Can you work these out from the model? Positions are in its coordinate system, mm. A direction names the side the tool comes from. Give positions to 0.01 mm unless a question says otherwise; leave off trailing zeros. Order: outer loops, then holes, each group sorted by start corner. A loop starts at its lowest first (then second) coordinate and runs counter-clockwise, first axis right, second up. Notation, with made-up numbers: (-28.5, -22.5) - (16.5, -22.5) arc R13 ccw to (16.5, -6.5) - close; hole circle Ø10 at (50.5, 32.5). An arc over 180 degrees is marked (long way). Answer as CSV lines item,"result".
```python
from build123d import *

# Parameters (mm, degrees)
SKETCH_1_R          = 1
EXTRUDE_1_DEPTH     = 4
SKETCH_2_W          = 15
SKETCH_2_H          = 4
CUT_EXTRUDE_1_DEPTH = 10
SKETCH_3_W          = 4
SKETCH_3_H          = 6.5
EXTRUDE_2_DEPTH     = 4


with BuildPart() as part:
    # Эскиз1 → Бобышка-Вытянуть1 (new body)
    with BuildSketch(Plane.XY):
        Polygon((0, 0), (0, 15), (3, 15), (3, 5), (22, 5), (22, 15), (49.5, 15), (49.5, -6), (0, -6), align=None)
        with Locations((22.5, 2)):
            Circle(SKETCH_1_R, mode=Mode.SUBTRACT)
        with Locations(Location((2, 2, 0), (0, 0, 180))):
            Circle(SKETCH_1_R, mode=Mode.SUBTRACT)
    extrude(amount=EXTRUDE_1_DEPTH)

    # Эскиз2 → Вырез-Вытянуть1 (cut)
    with BuildSketch(Plane.XY.offset(4)):
        with Locations((34.5, -4)):
            Rectangle(SKETCH_2_W, SKETCH_2_H)
    extrude(amount=-CUT_EXTRUDE_1_DEPTH, mode=Mode.SUBTRACT)

    # Эскиз3 → Бобышка-Вытянуть2 (add)
    with BuildSketch(Plane.XY.offset(4)):
        with Locations((-2, -2.75)):
            Rectangle(SKETCH_3_W, SKETCH_3_H)
        with Locations((-2, 11.75)):
            Rectangle(SKETCH_3_W, SKETCH_3_H)
        with Locations((51.5, 11.75)):
            Rectangle(SKETCH_3_W, SKETCH_3_H)
        with Locations((51.5, -2.75)):
            Rectangle(SKETCH_3_W, SKETCH_3_H)
    extrude(amount=-EXTRUDE_2_DEPTH)


solid = part.part
```
1) I want a section at A-A on x = 22.5. Write out the boundary of the cut face in (y, z).
Answer block:
outline,"(-6, 0) - (1, 0) - (1, 4) - (-6, 4) - close; (3, 0) - (15, 0) - (15, 4) - (3, 4) - close"
2) I need wall thicknesses on line 1 along Y through (x, z) = (22.5, 2); line 2 along X through (y, z) = (-4, 2.8); line 3 along X through (y, z) = (5.25, 3.5). Which ranges of each line are inside material? Lowest first, please. Write a range as [from, to].
Answer block:
line 1,"[-6, 1], [3, 15]"
line 2,"[-4, 27], [42, 53.5]"
line 3,"[0, 3], [22, 49.5]"
3) I'm going to push a flat-ended pin straight in: P1, Ø1.2, axis at x = 31.5, z = 2, coming from the -Y side. Where does the tip first touch, or does it pass through?
Answer block:
P1,"y = -2"
4) Which directions (+Z, -Z, +X, -X, +Y, -Y) give clear straight access to the entire face, cutting with the end or side of a thin tool? Please do faces 1 (the flat face through (22, 10, 2)), 2 (the flat face through (34, -2, 2)), 3 (the flat face through (51, 0.5, 2)), 4 (the flat face through (-2, 0.5, 2)).
Answer block:
face 1,"+Z, -Z, +Y"
face 2,"+Z, -Z, -Y"
face 3,"+Z, -Z, +X"
face 4,"+Z, -Z, -X"
5) If we mould it in two halves opening along X, with no side actions, what happens to faces 5 (the flat face through (48, -6, 2)), 6 (the flat face through (3, 10, 2)), 7 (the flat face through (-4, 12, 2))? For each: +X half, -X half, draft (parallel to the pull), parting line (faces both ways), or undercut.
Answer block:
face 5,"draft"
face 6,"undercut"
face 7,"-X half"
6) I want a section at D-D on z = 1.2. Write out the boundary of the cut face in (x, y).
Answer block:
outline,"(-4, -6) - (27, -6) - (27, -2) - (42, -2) - (42, -6) - (53.5, -6) - (53.5, 0.5) - (49.5, 0.5) - (49.5, 8.5) - (53.5, 8.5) - (53.5, 15) - (22, 15) - (22, 5) - (3, 5) - (3, 15) - (-4, 15) - (-4, 8.5) - (0, 8.5) - (0, 0.5) - (-4, 0.5) - close; hole circle Ø2 at (2, 2); hole circle Ø2 at (22.5, 2)"
7) I want a section at B-B on y = 2. Write out the boundary of the cut face in (x, z), plus the area to 3 significant figures.
Answer block:
outline,"(0, 0) - (1, 0) - (1, 4) - (0, 4) - close; (3, 0) - (21.5, 0) - (21.5, 4) - (3, 4) - close; (23.5, 0) - (49.5, 0) - (49.5, 4) - (23.5, 4) - close"
area,"182 mm2"
8) I want a section at C-C on y = -3. Write out the boundary of the cut face in (x, z), plus the area to 3 significant figures.
Answer block:
outline,"(-4, 0) - (27, 0) - (27, 4) - (-4, 4) - close; (42, 0) - (53.5, 0) - (53.5, 4) - (42, 4) - close"
area,"170 mm2"
